Work out the finished part from the listing and answer in its coordinate system (mm). Round coordinates to 2 decimals unless told otherwise and drop trailing zeros. Write each loop counter-clockwise with the first axis right and the second up, starting at its lowest first coordinate (ties: lowest second). Pieces come first, ordered by that corner, then holes. Notation, with made-up numbers: (79, 78) -> (93, 78) arc R19 ccw to (93, 107) -> close; hole circle Ø8 at (85.5, 3). An arc over 180 degrees is marked (long way). Answer as a JSON object with one key per item and string values. Group by question number.
from build123d import *

# Parameters (mm, degrees)
HEADSIDELEFT_THICKNESS_DEPTH      = 17.78
HEADSIDELEFTLEDGE_THICKNESS_DEPTH = 12.7
SKETCH4_W                         = 146.050000002
SKETCH4_H                         = 17.78
CUT_EXTRUDE2_DEPTH                = 5.08
SKETCH6_R                         = 3.302000001
SKETCH6_R_2                       = 3.302
CUT_EXTRUDE3_DEPTH                = 5.08
SKETCH3_R                         = 1.5875
CUT_EXTRUDE1_DEPTH                = 17.78


with BuildPart() as part:
    # HeadSideLeftOutline → HeadSideLeft_Thickness (new body)
    with BuildSketch(Plane.XY):
        Polygon((839.47, -5504.129603175), (839.47, -5314.95), (174.9425, -5314.95), (174.9425, -5573.445396825), align=None)
    extrude(amount=-HEADSIDELEFT_THICKNESS_DEPTH)

    # HeadSideLeftLedge → HeadSideLeftLedge_Thickness (add)
    with BuildSketch(Plane(origin=(0, 0, -17.78), x_dir=(-1, 0, 0), z_dir=(0, 0, -1))):
        Polygon((-174.9425, -5314.95), (-157.1625, -5314.95), (-157.1625, -5575.3), (-174.9425, -5573.445396825), align=None)
        Polygon((-839.47, -5314.95), (-857.25, -5314.95), (-857.25, -5502.275), (-839.47, -5504.129603175), align=None)
    extrude(amount=-HEADSIDELEFTLEDGE_THICKNESS_DEPTH)

    # Sketch4 → Cut-Extrude2 (cut)
    with BuildSketch(Plane.XY):
        with Locations((522.2875, -5417.566000001)):
            Rectangle(SKETCH4_W, SKETCH4_H)
    extrude(amount=-CUT_EXTRUDE2_DEPTH, mode=Mode.SUBTRACT)

    # Sketch6 → Cut-Extrude3 (cut)
    with BuildSketch(Plane.XY):
        with Locations((451.507564029, -5410.921064031)):
            Circle(SKETCH6_R)
        with Locations((451.507564029, -5424.210935971)):
            Circle(SKETCH6_R_2)
        with Locations((593.067435971, -5424.210935971)):
            Circle(SKETCH6_R_2)
        with Locations((593.067435971, -5410.921064031)):
            Circle(SKETCH6_R)
    extrude(amount=-CUT_EXTRUDE3_DEPTH, mode=Mode.SUBTRACT)

    # Sketch3 → Cut-Extrude1 (cut)
    with BuildSketch(Plane.XY):
        with Locations((166.0525, -5531.135582009)):
            Circle(SKETCH3_R)
        with Locations((166.0525, -5444.661349205)):
            Circle(SKETCH3_R)
        with Locations((166.0525, -5358.187116401)):
            Circle(SKETCH3_R)
        with Locations((848.36, -5471.826917991)):
            Circle(SKETCH3_R)
        with Locations((848.36, -5409.076150795)):
            Circle(SKETCH3_R)
        with Locations((848.36, -5346.325383599)):
            Circle(SKETCH3_R)
        with Locations((573.0875, -5417.566)):
            Circle(SKETCH3_R)
        with Locations((522.2875, -5417.566)):
            Circle(SKETCH3_R)
        with Locations((471.4875, -5417.566)):
            Circle(SKETCH3_R)
    extrude(amount=-CUT_EXTRUDE1_DEPTH, mode=Mode.SUBTRACT)


solid = part.part
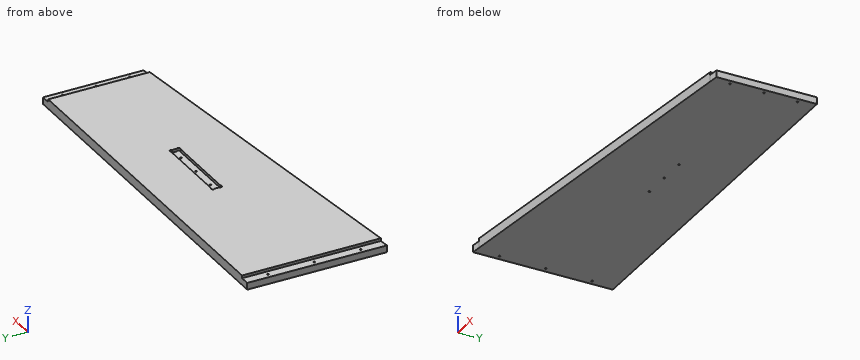
1) Each of these flat-tipped pins is pushed along its axis until it touches: P1, Ø2.5, axis at y = -5419, z = -1.5, coming from the -X side; P2, Ø5.5, axis at x = 851.5, y = -5378, coming from the +Z side; P3, Ø1, axis at y = -5387, z = -2, coming from the +X side. Where does it stop, or does it pass through?
2) A cutting plane is placed at B-B on x = 583. Determine the outline of the cut face in (y, z), plus the area to 3 significant figures.
3) A cutting plane is placed at D-D on x = 671. Determine the outline of the cut face in (y, z).
4) A cutting plane is placed at C-C on y = -5539. Determine the outline of the cut face in (x, z).
5) A cutting plane is placed at A-A on z = -9. State how many separate pieces and enclosed holes the cut face has, plus the area to 3 significant figures.
6) Straight lines are drawn through the part: L1, parallel to Y at x = 848.36, z = -11.5; L2, parallel to X at y = -5443.5, z = -0.75; L3, parallel to Y at x = 238.5, z = -4. For each, find the intervals that lie inside material, in ascending order.
Established:
{
 "1": {"P1": "stops at x = 174.94", "P2": "stops at z = -5.08", "P3": "stops at x = 839.47"},
 "2": {"outline": "(-5530.88, -17.78) -> (-5314.95, -17.78) -> (-5314.95, 0) -> (-5408.68, 0) -> (-5408.68, -5.08) -> (-5426.46, -5.08) -> (-5426.46, 0) -> (-5530.88, 0) -> close", "area": "3,750 mm²"},
 "3": {"outline": "(-5521.7, -17.78) -> (-5314.95, -17.78) -> (-5314.95, 0) -> (-5521.7, 0) -> close"},
 "4": {"outline": "(157.16, -17.78) -> (505.17, -17.78) -> (505.17, 0) -> (174.94, 0) -> (174.94, -5.08) -> (157.16, -5.08) -> close"},
 "5": {"separate pieces": "1", "enclosed holes": "9", "area": "157,000 mm²"},
 "6": {"L1": "y = -5503.2 to -5473.41, -5470.24 to -5410.66, -5407.49 to -5347.91, -5344.74 to -5314.95", "L2": "x = 174.94 to 839.47", "L3": "y = -5566.82 to -5314.95"}
}
